from build123d import *

# Parameters (mm, degrees)
F0_R     = 4
F1_DEPTH = 5


with BuildPart() as f1:
    # F0 (on Front) → F1 (new body)
    with BuildSketch(Plane.XZ):
        with BuildLine():
            ThreePointArc((-162.93692, 35.030597), (-158.898512, 38.999814), (-154.937307, 34.953548))
            Line((-154.937307, 34.953548), (-154.940273, 34.69815))
            ThreePointArc((-154.940273, 34.69815), (-152.941566, 29.718719), (-148.004667, 27.617152))
            Line((-148.004667, 27.617152), (-122.802143, 27.387))
            ThreePointArc((-122.802143, 27.387), (-120.179499, 26.522977), (-118.415412, 24.398643))
            Line((-118.415412, 24.398643), (-110.784866, 6.997219))
            ThreePointArc((-110.784866, 6.997219), (-104.156475, 2.525958), (-97.277175, 6.600632))
            Line((-97.277175, 6.600632), (-88.737962, 23.330208))
            ThreePointArc((-88.737962, 23.330208), (-86.812994, 25.370653), (-84.092183, 26.05337))
            Line((-84.092183, 26.05337), (-60.199575, 25.133445))
            ThreePointArc((-60.199575, 25.133445), (-55.076662, 27.084195), (-52.930257, 32.128262))
            Line((-52.930257, 32.128262), (-52.930257, 34.767204))
            ThreePointArc((-52.930257, 34.767204), (-52.937037, 35), (-52.930257, 35.232796))
            ThreePointArc((-52.930257, 35.232796), (-48.82609, 38.998461), (-44.937052, 35.011005))
            Line((-44.937052, 35.011005), (-44.650559, 32.005813))
            ThreePointArc((-44.650559, 32.005813), (-42.052043, 28.082513), (-37.346324, 28.054719))
            Line((-37.346324, 28.054719), (-11.957943, 41.402887))
            ThreePointArc((-11.957943, 41.402887), (-9.223694, 43.979528), (-8.215466, 47.598736))
            Line((-8.215466, 47.598736), (-8.215466, 76.367726))
            ThreePointArc((-8.215466, 76.367726), (-10.265719, 81.317474), (-15.215466, 83.367726))
            Line((-15.215466, 83.367726), (-191.405466, 83.367726))
            ThreePointArc((-191.405466, 83.367726), (-196.355214, 81.317474), (-198.405466, 76.367726))
            Line((-198.405466, 76.367726), (-198.405466, 48.917622))
            ThreePointArc((-198.405466, 48.917622), (-197.494704, 45.464917), (-194.999416, 42.910666))
            Line((-194.999416, 42.910666), (-172.017448, 29.160603))
            ThreePointArc((-172.017448, 29.160603), (-165.977458, 29.090075), (-162.93692, 34.309423))
            Line((-162.93692, 34.309423), (-162.93692, 34.969403))
            ThreePointArc((-162.93692, 34.969403), (-162.937037, 35), (-162.93692, 35.030597))
        make_face()
        with BuildLine():
            ThreePointArc((-100.937777, 9.933366), (-106.936852, 10.033319), (-100.937037, 10))
            ThreePointArc((-100.937037, 10), (-100.937051, 9.990837), (-100.937093, 9.981674))
            Line((-100.937093, 9.981674), (-100.937777, 9.933366))
        make_face(mode=Mode.SUBTRACT)
        with BuildLine():
            ThreePointArc((-189.357673, 58.750004), (-187.33795, 61.585327), (-183.998301, 60.602938))
            Line((-183.998301, 60.602938), (-169.280903, 41.863033))
            ThreePointArc((-169.280903, 41.863033), (-169.389036, 38.027191), (-173.180539, 37.435689))
            Line((-173.180539, 37.435689), (-187.897937, 46.241077))
            ThreePointArc((-187.897937, 46.241077), (-188.967347, 47.335756), (-189.357673, 48.815487))
            Line((-189.357673, 48.815487), (-189.357673, 58.750004))
        make_face(mode=Mode.SUBTRACT)
        with BuildLine():
            Line((-144.227608, 40.453975), (-112.364396, 62.860901))
            ThreePointArc((-112.364396, 62.860901), (-109.274696, 63.078906), (-107.638996, 60.448647))
            Line((-107.638996, 60.448647), (-107.327348, 38.041722))
            ThreePointArc((-107.327348, 38.041722), (-108.191037, 35.893482), (-110.327057, 35))
            Line((-110.327057, 35), (-142.501918, 35))
            ThreePointArc((-142.501918, 35), (-145.362156, 37.094993), (-144.227608, 40.453975))
        make_face(mode=Mode.SUBTRACT)
        with BuildLine():
            Line((-158.161986, 46.343195), (-178.982052, 67.12042))
            ThreePointArc((-178.982052, 67.12042), (-180.288218, 73.660732), (-174.743657, 77.367428))
            Line((-174.743657, 77.367428), (-124.237035, 77.366367))
            ThreePointArc((-124.237035, 77.366367), (-118.514624, 73.169857), (-120.796878, 66.450631))
            Line((-120.796878, 66.450631), (-150.483435, 45.674467))
            ThreePointArc((-150.483435, 45.674467), (-154.444289, 44.612828), (-158.161986, 46.343195))
        make_face(mode=Mode.SUBTRACT)
        with Locations((-188.937037, 73.367726)):
            Circle(F0_R, mode=Mode.SUBTRACT)
        with BuildLine():
            ThreePointArc((-100.027452, 74.213391), (-99.959705, 73.792969), (-99.937037, 73.367726))
            ThreePointArc((-99.937037, 73.367726), (-99.966125, 72.886206), (-100.052968, 72.411689))
            ThreePointArc((-100.052968, 72.411689), (-103.9034, 69.367868), (-107.804478, 72.346502))
            ThreePointArc((-107.804478, 72.346502), (-107.93665, 73.312097), (-107.831384, 74.280995))
            ThreePointArc((-107.831384, 74.280995), (-103.902387, 77.367576), (-100.027452, 74.213391))
        make_face(mode=Mode.SUBTRACT)
        with BuildLine():
            ThreePointArc((-100.222687, 60.427463), (-98.585652, 63.057648), (-95.495448, 62.837655))
            Line((-95.495448, 62.837655), (-63.714392, 40.452673))
            ThreePointArc((-63.714392, 40.452673), (-62.582035, 37.093915), (-65.441931, 35))
            Line((-65.441931, 35), (-97.540001, 35))
            ThreePointArc((-97.540001, 35), (-99.676288, 35.893753), (-100.5397, 38.042481))
            Line((-100.5397, 38.042481), (-100.222687, 60.427463))
        make_face(mode=Mode.SUBTRACT)
        with BuildLine():
            Line((-59.062029, 46.891406), (-89.817697, 68.225334))
            ThreePointArc((-89.817697, 68.225334), (-91.738656, 73.830314), (-86.960347, 77.333691))
            Line((-86.960347, 77.333691), (-33.232048, 77.252552))
            ThreePointArc((-33.232048, 77.252552), (-27.844669, 73.875237), (-28.517809, 67.552501))
            Line((-28.517809, 67.552501), (-42.775908, 49.351358))
            ThreePointArc((-42.775908, 49.351358), (-50.430287, 44.886066), (-59.062029, 46.891406))
        make_face(mode=Mode.SUBTRACT)
        with BuildLine():
            Line((-37.495455, 43.158397), (-20.822425, 64.520861))
            ThreePointArc((-20.822425, 64.520861), (-17.481474, 65.511855), (-15.457471, 62.675056))
            Line((-15.457471, 62.675056), (-15.457471, 50.078587))
            ThreePointArc((-15.457471, 50.078587), (-15.889569, 48.527498), (-17.06139, 47.423223))
            Line((-17.06139, 47.423223), (-33.73442, 38.657229))
            ThreePointArc((-33.73442, 38.657229), (-37.432632, 39.389004), (-37.495455, 43.158397))
        make_face(mode=Mode.SUBTRACT)
        with Locations((-18.937037, 73.367726)):
            Circle(F0_R, mode=Mode.SUBTRACT)
    extrude(amount=F1_DEPTH)


solid = f1.part
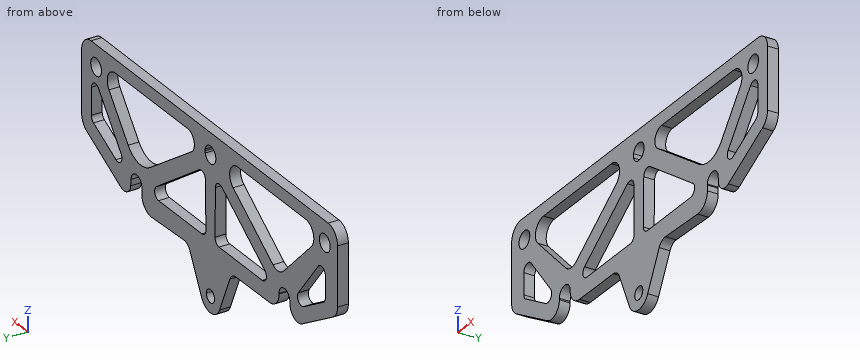
The listing builds one solid part. Answer for the finished solid, in the listing's coordinates (mm). Coordinates: 2 decimals unless noted, no trailing zeros. Order: outer loops, then holes, each group sorted by start corner. A loop starts at its lowest first (then second) coordinate and runs counter-clockwise, first axis right, second up. Notation, with made-up numbers: M -13.5,7 L -2.5,7 A19 ccw -2.5,26 Z; hole C -4.5,57.25 d2. An arc over 180 degrees is marked long. Use CSV: the item, a comma, the result in double quotes.
Q1. Given pin 1 Ø1.5 at (x, y) = (-126.5, -1) entering from -Z; pin 2 Ø0.8 at (y, z) = (-3.5, 33.5) entering from +X; pin 3 Ø2.5 at (x, y) = (-152.5, -2.5) entering from -Z, each flat-ended and moving along its own axis, determine where each tip first touches the part or whether it passes through.
Here are the results:
pin 1,"z = 27.41"
pin 2,"x = -26.23"
pin 3,"z = 28.45"
Q2. Section A-A (x = -126) is taken. Determine the outline of the cut face in (y, z).
Here are the results:
outline,"M -5,27.42 L 0,27.42 L 0,35 L -5,35 Z; M -5,53.27 L 0,53.27 L 0,62.81 L -5,62.81 Z; M -5,77.37 L 0,77.37 L 0,83.37 L -5,83.37 Z"
Q3. Section B-B (y = -3.65) is taken. Give the number of separate pieces and of enclosed holes in the cut face, then the cut area to 3 significant figures.
Here are the results:
separate pieces,"1"
enclosed holes,"10"
area,"5,670 mm2"
Q4. Straight lines are drawn through the part: L1, parallel to Z at x = -169.5, y = -2.7; L2, parallel to X at y = -1.45, z = 34.5; L3, parallel to Z at x = -66, y = -4. For each, find the intervals that lie inside material, in ascending order.
Here are the results:
L1,"28.34 to 37.91, 42.14 to 57.66, 77.37 to 83.37"
L2,"-180.94 to -162.94, -154.94 to -52.93, -44.89 to -25.09"
L3,"25.36 to 35, 42.06 to 51.7, 77.3 to 83.37"
Q5. Section C-C (z = 19) is taken. Determine the outline of the cut face in (x, y).
Here are the results:
outline,"M -116.05,-5 L -90.95,-5 L -90.95,0 L -116.05,0 Z"
